Verification items for the finished model (mm, model axes). A direction names the side the tool comes from. Give positions to 0.01 mm unless a question says otherwise; leave off trailing zeros. Order: outer loops, then holes, each group sorted by start corner. A loop starts at its lowest first (then second) coordinate and runs counter-clockwise, first axis right, second up.
(1) Sectioned sample at D-D on x = 43.5. Record the cut outline in (y, z).
(2) Mould release check, pull along X, two halves, no side actions. Record for faces 1 (the face through (59.29, -18, 19)), 2 (the face through (64.543, -15.53, 19.338)), 3 (the face through (66, -31.5, 19)): pulls with the +X half, pulls with the -X half, needs draft (parallel to the pull), parting line crosses it, or undercut.
(3) Access from +Z, -Z, +X, -X, +Y, -Y to the whole of each face (thin tool, end or side, straight path). Record for faces 4 (the face through (-11, -2, 17)), 5 (the face through (66, -18, 12.95)), 6 (the face through (38.971, -2.465, -13.626)), 7 (the face through (59.29, -2, 28)).
(4) Sectioned sample at A-A on z = -12. Record the cut outline in (x, y).
(5) Sectioned sample at C-C on z = 14.5. Record the cut outline in (x, y), plus the area to 3 significant figures.
(6) Sectioned sample at B-B on y = -23.5. Record the cut outline in (x, z).
(7) Gauge pin test, flat ends, axial feed: pin 1 (1.5 mm diameter, centred on x = -2, z = -22.5, fed in from -Y); pin 2 (6 mm diameter, centred on y = -3.5, z = 9.5, fed in from +X) (3 decimals); pin 3 (6 mm diameter, centred on x = 19, y = -9, fed in from +Z); pin 4 (9.5 mm diameter, centred on y = -18, z = 20.5, fed in from -X). Record the tip position at first contact, or that the pin passes through.
(8) Scan lines: L1, parallel to Y at x = 28, z = 25; L2, parallel to Z at x = 67, y = -26; L3, parallel to X at y = -2.5, z = -3. Record each from-to range of solid material in increasing order.
```python
from build123d import *

# Parameters (mm, degrees)
F1_DEPTH = 5
F0_W     = 14.0000022948
F0_H     = 11.7600001395
F0_R     = 1.6916232852
F0_R_2   = 1.7089194305
F7_DEPTH = 31.5
F8_DEPTH = 2


# Not quite as in the source:
# - the program builds the solid bodies; features that only make, move or delete a surface that nothing else refers to are left out


with BuildPart() as f1:
    # F0 (on Front) → F1 (new body)
    with BuildSketch(Plane.XZ):
        with BuildLine():
            ThreePointArc((0, -25), (-25, 0), (0, 25))
            Line((0, 25), (0, 31.0474538393))
            ThreePointArc((0, 31.0474538393), (-29.8919830792, 0.5977015918), (0, -29.8520506557))
            Line((0, -29.8520506557), (0, -25))
        make_face()
        with BuildLine():
            ThreePointArc((0, 25), (17.6776695297, 17.6776695297), (25, 0))
            ThreePointArc((25, 0), (17.6776695297, -17.6776695297), (0, -25))
            Line((0, -25), (0, -29.8520506557))
            ThreePointArc((0, -29.8520506557), (39.4905936266, -13.3235446474), (73.2899941504, 12.9499975592))
            Line((73.2899941504, 12.9499975592), (59.2899918556, 12.9499975592))
            Line((59.2899918556, 12.9499975592), (59.2899918556, 24.7099976987))
            Line((59.2899918556, 24.7099976987), (59.2899918556, 31.0100000352))
            Line((59.2899918556, 31.0100000352), (0, 31.0474538393))
            Line((0, 31.0474538393), (0, 25))
        make_face()
    extrude(amount=F1_DEPTH)

    # F0 (on Front) → F7 (join)
    with BuildSketch(Plane.XZ):
        with Locations((66.289993003, 18.8299976289)):
            Rectangle(F0_W, F0_H)
        with Locations((62.9299916327, 18.8299976289)):
            Circle(F0_R, mode=Mode.SUBTRACT)
        with Locations((69.9299909174, 18.8299976289)):
            Circle(F0_R_2, mode=Mode.SUBTRACT)
    extrude(amount=F7_DEPTH)

    # F0 (on Front) → F8 (join)
    with BuildSketch(Plane.XZ):
        with BuildLine():
            ThreePointArc((0, -25), (17.6776695297, -17.6776695297), (25, 0))
            ThreePointArc((25, 0), (17.6776695297, 17.6776695297), (0, 25))
            Line((0, 25), (0, 20))
            ThreePointArc((0, 20), (14.1421356237, 14.1421356237), (20, 0))
            ThreePointArc((20, 0), (14.1421356237, -14.1421356237), (0, -20))
            Line((0, -20), (0, -25))
        make_face()
        with BuildLine():
            Line((0, 20), (0, 25))
            ThreePointArc((0, 25), (-25, 0), (0, -25))
            Line((0, -25), (0, -20))
            ThreePointArc((0, -20), (-20, 0), (0, 20))
        make_face()
    extrude(amount=F8_DEPTH)


solid = f1.part
```
Ans:
1. outline: (-5, -10.9) - (0, -10.9) - (0, 31.02) - (-5, 31.02) - close
2. face 1: pulls with the -X half
2. face 2: undercut
2. face 3: needs draft
3. face 4: -Y
3. face 5: -Z, +X, -X, -Y
3. face 6: -Z, +X, +Y, -Y
3. face 7: +Z, +X, +Y, -Y
4. outline: (-27.16, -5) - (-21.93, -5) - (-21.93, -2) - (-16, -2) - (-16, 0) - (-27.16, 0) - close; (16, -2) - (21.93, -2) - (21.93, -5) - (41.72, -5) - (41.72, 0) - (16, 0) - close
5. outline: (-26.53, -5) - (-20.37, -5) - (-20.37, -2) - (-13.77, -2) - (-13.77, 0) - (-26.53, 0) - close; (13.77, -2) - (20.37, -2) - (20.37, -5) - (59.29, -5) - (59.29, -31.5) - (73.29, -31.5) - (73.29, 0) - (13.77, 0) - close
5. area: 693 mm2
6. outline: (59.29, 12.95) - (73.29, 12.95) - (73.29, 24.71) - (59.29, 24.71) - close; hole circle Ø3.38 at (62.93, 18.83); hole circle Ø3.42 at (69.93, 18.83)
7. pin 1: stops at y = -2
7. pin 2: stops at x = 72.845
7. pin 3: passes through
7. pin 4: stops at x = 59.29
8. L1: y = -5 to 0
8. L2: z = 12.95 to 24.71
8. L3: x = -29.68 to -24.82, 24.82 to 55.04
